Input: dimensioned drawing with shaded views. Units: mm. Origin: part minimum x, y, z. A direction names the side the tool comes from. Round coordinates to 2 decimals unless told otherwise and drop trailing zeros. Order: outer loops, then holes, each group sorted by start corner. A loop starts at its lowest first (then second) coordinate and runs counter-clockwise, first axis right, second up. Notation, with made-up numbers: M -38.75,-3.75 L -6.75,-3.75 A32 cw -6.75,22.25 Z; hole C -36.5,55 d3. An arc over 180 degrees is marked long. Use one line per item in the form item = value. Start each with the question number.
Q1. Reachability of the marked faces 4 and 5 from +Z, -Z, +X, -X, +Y, -Y: full face, straight path, thin tool, end or side. Return the list, or none.
Q2. Material intervals for probe 1 along X at (y, z) = (37, 75); probe 2 along X at (y, z) = (8, 75); probe 3 along Z at (x, y) = (81.5, 16), sorted ascending.
Q3. Section B-B (x = 75). Return the cut outline in (y, z).
Q4. Section C-C (y = 48). Return the cut outline in (x, z).
Q5. Section D-D (y = 4.5). Return the cut outline in (x, z).
Q6. Pull-direction query (X, two-part tool) for the marked faces 1, 2 and 3; classes: pulls with the +X half, pulls with the -X half, needs draft (parallel to the pull), parting line crosses it, or undercut.
Q7. Contact query for flat-ended pins moving along their axis: pin 1 (10 mm diameter, centred on x = 108, y = 36.5, fed in from -Z); pin 2 (2 mm diameter, centred on y = 35, z = 30, fed in from -X); pin 3 (10 mm diameter, centred on y = 51.5, z = 92, fed in from -X). Output: stop coordinate, or through.
Q8. Section A-A (z = 75). Return the cut outline in (x, y).
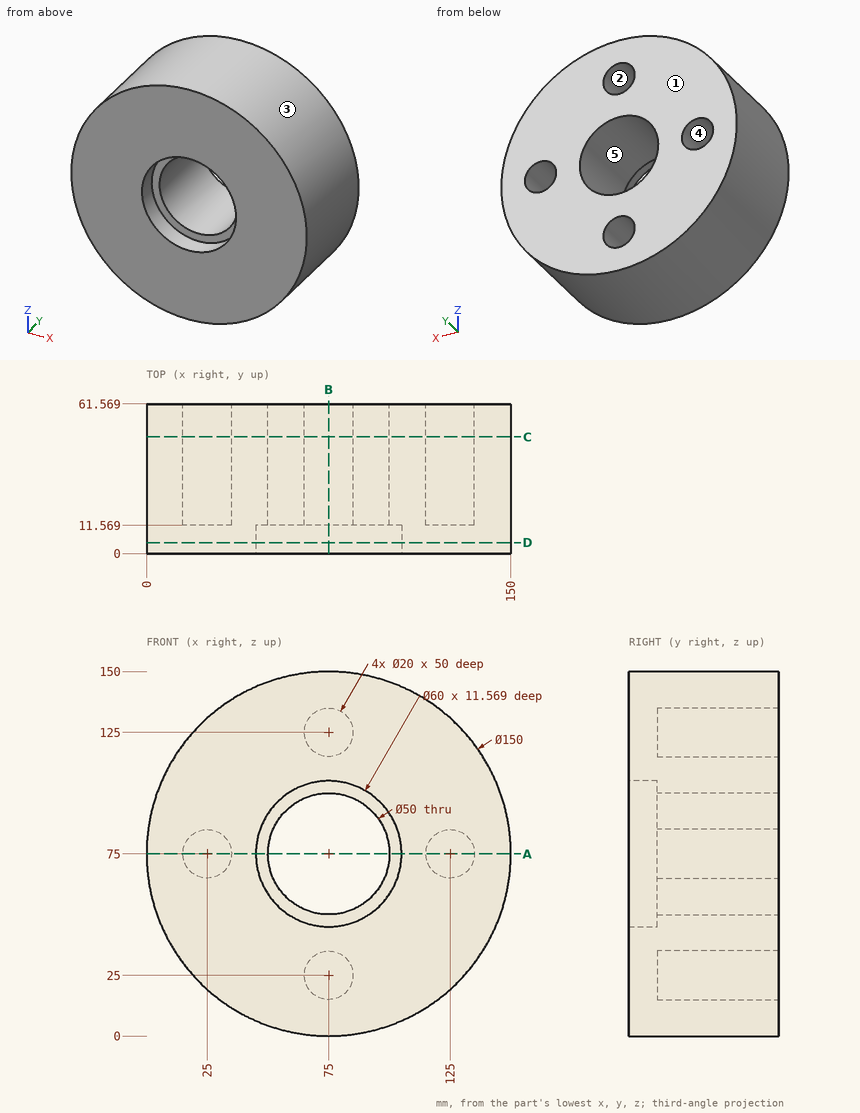
Results list:
q1.face_4 = +Y
q1.face_5 = +Y, -Y
q2.probe_1 = 0 to 15, 35 to 50, 100 to 115, 135 to 150
q2.probe_2 = 0 to 45, 105 to 150
q2.probe_3 = 0.28 to 17.4, 32.6 to 50.86, 99.14 to 117.4, 132.6 to 149.72
q3.outline = M 0,0 L 61.57,0 L 61.57,15 L 11.57,15 L 11.57,35 L 61.57,35 L 61.57,50 L 11.57,50 L 11.57,45 L 0,45 Z; M 0,105 L 11.57,105 L 11.57,100 L 61.57,100 L 61.57,115 L 11.57,115 L 11.57,135 L 61.57,135 L 61.57,150 L 0,150 Z
q4.outline = C 75,75 d150; hole C 25,75 d20; hole C 75,75 d50; hole C 75,25 d20; hole C 75,125 d20; hole C 125,75 d20
q5.outline = C 75,75 d150; hole C 75,75 d60
q6.face_1 = needs draft
q6.face_2 = undercut
q6.face_3 = parting line crosses it
q7.pin_1 = 5.42
q7.pin_2 = 14.26
q7.pin_3 = 0.97
q8.outline = M 0,0 L 45,0 L 45,11.57 L 50,11.57 L 50,61.57 L 35,61.57 L 35,11.57 L 15,11.57 L 15,61.57 L 0,61.57 Z; M 100,11.57 L 105,11.57 L 105,0 L 150,0 L 150,61.57 L 135,61.57 L 135,11.57 L 115,11.57 L 115,61.57 L 100,61.57 Z
